Here's how the part is built. I have some questions about the finished solid (model axes, mm). Round coordinates to 2 decimals unless told otherwise and drop trailing zeros. Loops run counter-clockwise (first coordinate to the right, second up) from the corner with the lowest first, then second, coordinate; pieces in that order, holes last. Notation, with made-up numbers: (11.25, 68) - (53.25, 68) arc R26 ccw to (53.25, 94) - close; hole circle Ø11 at (5, 63). An arc over 180 degrees is marked (long way). Answer as a JSON object with one key per item and string values. Group by question number.
1) I want a section at C-C, the plane z = -6.95. Please give me the cut outline in (x, y).
2) If I drill on line 1 along X through (y, z) = (-8, 5.75); line 2 along Z through (x, y) = (-2.25, -13.5); line 3 along X through (y, z) = (-13, 2), over which ranges is the centre line in solid material (lowest first)? Write a range as [from, to].
3) Will these pins go through, and if not, where does the flat tip stop? P1, Ø5, axis at y = -8.5, z = 6.5, coming from the -X side; P2, Ø4, axis at y = -39, z = 3, coming from the -X side; P3, Ø12, axis at y = -9.5, z = 8, coming from the +X side.
4) I want a section at B-B, the plane x = 0.25. Please give me the cut outline in (y, z).
5) I want a section at A-A, the plane z = 0. Please give me the cut outline in (x, y) (3 decimals), then the cut area to 3 significant figures.
6) If we mould it in two halves opening along X, with no side actions, what happens to faces 1 (the face through (4.34, -10.52, -7.6)), 2 (the face through (6, -47.8, 4)), 3 (the face through (12.09, -10.52, 3.81))? For each: pulls with the +X half, pulls with the -X half, needs draft (parallel to the pull), parting line crosses it, or undercut.
7) I want a section at D-D, the plane y = -40. Please give me the cut outline in (x, z) (3 decimals), then the cut area to 3 significant figures.
from build123d import *

# Parameters (mm, degrees)
F0_R     = 2.5
F1_DEPTH = 47.8
F3_R     = 12.675
F3_R_2   = 8.75
F4_DEPTH = 11.2


with BuildPart() as f1:
    # F0 (on Front) → F1 (new body)
    with BuildSketch(Plane.XZ):
        with Locations((0, 6.95)):
            Circle(F0_R)
        with Locations((-6.018877, 3.475)):
            Circle(F0_R)
        with Locations((-6.018877, -3.475)):
            Circle(F0_R)
        with Locations((0, -6.95)):
            Circle(F0_R)
        with Locations((6.018877, -3.475)):
            Circle(F0_R)
        with Locations((6.018877, 3.475)):
            Circle(F0_R)
    extrude(amount=F1_DEPTH)

    # F3 (on offset) → F4 (join)
    with BuildSketch(Plane.XZ.offset(5)):
        Circle(F3_R)
        Circle(F3_R_2, mode=Mode.SUBTRACT)
    extrude(amount=F4_DEPTH)


solid = f1.part
Outcome:
{
 "1": {"outline": "(-10.6, -16.2) - (-5.32, -16.2) - (-5.32, -5) - (-10.6, -5) - close; (-2.5, -47.8) - (2.5, -47.8) - (2.5, 0) - (-2.5, 0) - close; (5.32, -16.2) - (10.6, -16.2) - (10.6, -5) - (5.32, -5) - close"},
 "2": {"line 1": "[-11.3, -4.98], [-2.19, 2.19], [4.98, 11.3]", "line 2": "[-12.47, -8.46], [-8.04, -5.86], [5.86, 8.04], [8.46, 12.47]", "line 3": "[-12.52, -8.52], [-8.04, -4], [4, 8.04], [8.52, 12.52]"},
 "3": {"P1": "x = -12.03", "P2": "x = -8.52", "P3": "x = 12.52"},
 "4": {"outline": "(-47.8, -9.44) - (-16.2, -9.44) - (-16.2, -12.67) - (-5, -12.67) - (-5, -9.44) - (0, -9.44) - (0, -4.46) - (-47.8, -4.46) - close; (-47.8, 4.46) - (0, 4.46) - (0, 9.44) - (-5, 9.44) - (-5, 12.67) - (-16.2, 12.67) - (-16.2, 9.44) - (-47.8, 9.44) - close"},
 "5": {"outline": "(-12.675, -16.2) - (-8.75, -16.2) - (-8.75, -5) - (-12.675, -5) - close; (8.75, -16.2) - (12.675, -16.2) - (12.675, -5) - (8.75, -5) - close", "area": "87.9 mm^2"},
 "6": {"face 1": "undercut", "face 2": "needs draft", "face 3": "parting line crosses it"},
 "7": {"outline": "circle Ø5 at (-6.019, -3.475); circle Ø5 at (-6.019, 3.475); circle Ø5 at (0, -6.95); circle Ø5 at (0, 6.95); circle Ø5 at (6.019, -3.475); circle Ø5 at (6.019, 3.475)", "area": "118 mm^2"}
}
